Part print with two shaded views. Sizes in mm from the minimum x, y, z corner. Round coordinates to 2 decimals unless told otherwise and drop trailing zeros. Loops run counter-clockwise (first coordinate to the right, second up) from the corner with the lowest first, then second, coordinate; pieces in that order, holes last. Notation, with made-up numbers: (46, 20) -> (88, 20) arc R26 cw to (88, 58) -> close; hole circle Ø9 at (17.5, 8.5). An arc over 180 degrees is marked (long way). Answer as a JSON object with one key per item and string values. Group by question number.
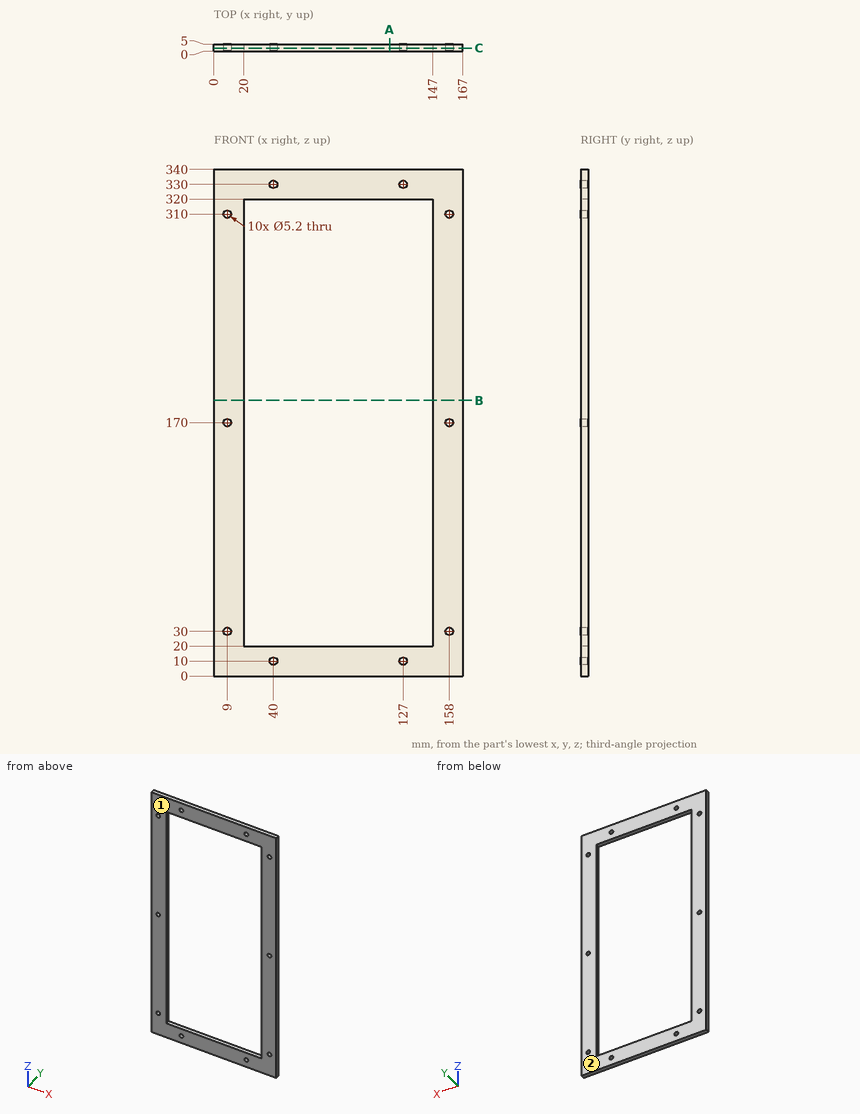
Item 1: Band-saw the part on B-B, the plane z = 185. List the corners of the cut face in (x, y).
Item 2: Drop a flat-ended pin along its axis: pin 1 Ø4.5 at (x, z) = (127, 330) entering from +Y. Give the stop position or say it passes through.
Item 3: Two-plate mould, pull along Y, no slides. Class the marked faces 1 and 2: pulls with the +Y half, pulls with the -Y half, needs draft (parallel to the pull), parting line crosses it, or undercut.
Item 4: Drill centre lines: line 1 (X direction, y = 2.25, z = 30); line 2 (Z direction, x = 158, y = 2.95); line 3 (X direction, y = 2.8, z = 176). Where is each one in solid material? Low to high.
Item 5: Band-saw the part on C-C, the plane y = 2.3. Count the separate pieces of the cut face and the enclosed holes in it, plus the area to 3 significant figures.
Item 6: Band-saw the part on A-A, the plane x = 118. List the corners of the cut face in (y, z).
Entries:
{
 "1": {"outline": "(0, 0) -> (20, 0) -> (20, 5) -> (0, 5) -> close; (147, 0) -> (167, 0) -> (167, 5) -> (147, 5) -> close"},
 "2": {"pin 1": "through"},
 "3": {"face 1": "pulls with the -Y half", "face 2": "pulls with the +Y half"},
 "4": {"line 1": "0 to 6.4, 11.6 to 20, 147 to 155.4, 160.6 to 167", "line 2": "0 to 27.4, 32.6 to 167.4, 172.6 to 307.4, 312.6 to 340", "line 3": "0 to 20, 147 to 167"},
 "5": {"separate pieces": "1", "enclosed holes": "11", "area": "18,500 mm²"},
 "6": {"outline": "(0, 0) -> (5, 0) -> (5, 20) -> (0, 20) -> close; (0, 320) -> (5, 320) -> (5, 340) -> (0, 340) -> close"}
}
